```python
from build123d import *

# Parameters (mm, degrees)
F0_R     = 3.96875
F1_DEPTH = 22.86
F2_R     = 7.62
F2_R_2   = 3.96875
F3_DEPTH = 17.78
F4_SIZE2 = 13.1982271537
F4_SIZE  = 7.62


with BuildPart() as f1:
    # F0 (on Top) → F1 (new body)
    with BuildSketch(Plane.XY):
        Circle(F0_R)
    extrude(amount=F1_DEPTH)

    # F2 (on face) → F3 (join)
    with BuildSketch(Plane.XY.offset(22.86)):
        Circle(F2_R)
        Circle(F2_R_2, mode=Mode.SUBTRACT)
        Circle(F2_R_2)
    extrude(amount=F3_DEPTH)

    # F4
    f4_edges = [f1.edges().sort_by_distance(p)[0] for p in [
        (-7.62, 0, 40.64),
    ]]
    f4_side = f1.faces().sort_by_distance((0, 0, 40.64))[0]
    chamfer(f4_edges, length=F4_SIZE, length2=F4_SIZE2, reference=f4_side)


solid = f1.part
```
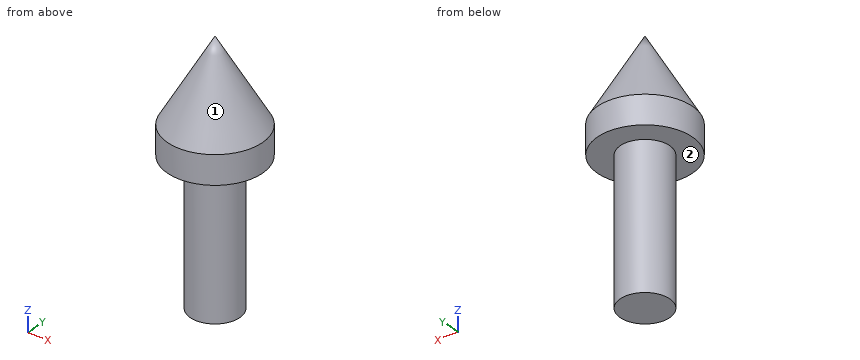
Geometry: final body of the model. Coordinates: model frame, mm. Face numbers are marked on the shaded views. A direction names the side the tool comes from. Give positions to 0.01 mm unless a question says otherwise; leave off trailing zeros. Write each loop counter-clockwise with the first axis right and the second up, starting at its lowest first coordinate (ties: lowest second). Pieces come first, ordered by that corner, then holes.
1. Pin query (flat end, axial travel): P1, Ø3, axis at y = 4, z = 30.5, coming from the -X side; P2, Ø6, axis at y = -3, z = 16.5, coming from the -X side; P3, Ø4, axis at x = 4, z = 22.5, coming from the -Y side; P4, Ø1.5, axis at x = 6, z = 10.5, coming from the +Y side. Return the tip coordinate at first contact, or that it passes through.
2. Section query B-B, the plane z = 37. Return loops of the section in (x, y).
3. Reachability of the marked faces 1 and 2 from +Z, -Z, +X, -X, +Y, -Y: full face, straight path, thin tool, end or side. Return the list, or none.
4. Section query A-A, the plane z = 15. Return loops of the section in (x, y).
5. Line query: probe 1 along X at (y, z) = (-0.75, 7); probe 2 along Y at (x, z) = (1.5, 17); probe 3 along X at (y, z) = (2.5, 16). Output: solid intervals per line, ascending.
Computed:
1. P1: stops at x = -5.77
1. P2: stops at x = -3.97
1. P3: stops at y = -7.34
1. P4: passes through
2. outline: circle Ø4.2 at (0, 0)
3. face 1: +Z
3. face 2: -Z
4. outline: circle Ø7.94 at (0, 0)
5. probe 1: x = -3.9 to 3.9
5. probe 2: y = -3.67 to 3.67
5. probe 3: x = -3.08 to 3.08
